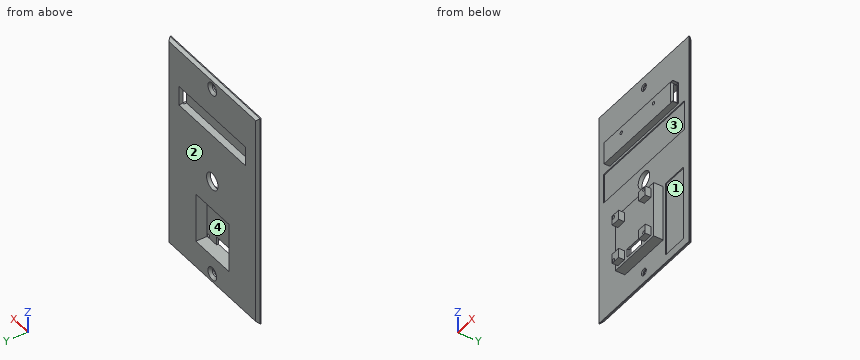
from build123d import *
from OCP.BRepFilletAPI import BRepFilletAPI_MakeChamfer

# Parameters (mm, degrees)
SKETCH2_W                = 69.35
SKETCH2_H                = 113.5
SKETCH2_R                = 1.85
BOSS_EXTRUDE3_DEPTH      = 2
SKETCH4_W                = 25.4
SKETCH4_H                = 26.1
CUT_EXTRUDE7_DEPTH       = 7.5
SKETCH16_W               = 29.414133621
SKETCH16_H               = 29.490350257
BOSS_EXTRUDE18_DEPTH     = 5
SKETCH17_W               = 25.4
SKETCH17_H               = 26.1
CUT_EXTRUDE8_DEPTH       = 4
SKETCH18_W               = 5
SKETCH18_H               = 5
BOSS_EXTRUDE24_DEPTH     = 4
SKETCH20_R               = 0.875
CUT_EXTRUDE10_DEPTH      = 4
SKETCH24_W               = 11
SKETCH24_H               = 4.5
CUT_EXTRUDE11_DEPTH      = 4
CHAMFER1_SIZE            = 1.5
CHAMFER1_SIZE2           = 1.258649447
SKETCH25_R               = 4.4
CUT_EXTRUDE12_DEPTH      = 4
SKETCH26_W               = 51.2
SKETCH26_H               = 10.3
CUT_EXTRUDE13_DEPTH      = 4
SKETCH27_W               = 52.651978828
SKETCH27_H               = 11.660574528
BOSS_EXTRUDE30_DEPTH     = 3
SKETCH30_W               = 51.2
SKETCH30_H               = 10.3
CUT_EXTRUDE14_DEPTH      = 3
SKETCH31_W               = 51.2
SKETCH31_H               = 10.3
BOSS_EXTRUDE31_DEPTH     = 1.5
SKETCH32_W               = 11.249454003
SKETCH32_H               = 2.603694337
CUT_EXTRUDE15_DEPTH      = 1.5
SKETCH33_W               = 1.5
SKETCH33_H               = 11.249454003
CUT_EXTRUDE16_DEPTH      = 1.5
SKETCH34_R               = 0.991075147
CUT_EXTRUDE17_DEPTH      = 1.5
SKETCH35_W               = 4.49763683
SKETCH35_H               = 1.113144729
CUT_EXTRUDE18_DEPTH      = 1.5
SKETCH36_W               = 62.277737466
SKETCH36_H               = 15.843958398
CUT_EXTRUDE19_DEPTH      = 0.5
SKETCH37_W               = 13.804637021
SKETCH37_H               = 39.531460558
CUT_EXTRUDE22_DEPTH      = 0.5
CHAMFER2_SIZE            = 1.5
CHAMFER2_SIZE2           = 1.258649447
CHAMFER3_SIZE            = 1.5
CHAMFER3_SIZE2           = 1.258649447
CUT_EXTRUDE23_DEPTH      = 67.821913509
CUT_EXTRUDE23_DEPTH_BACK = 67.821913509
SKETCH42_R               = 0.875


with BuildPart() as part:
    # Sketch2 → Boss-Extrude3 (new body)
    with BuildSketch(Plane(origin=(0, 0, 0), x_dir=(1, 0, 0), z_dir=(0, 1, 0))):
        Rectangle(SKETCH2_W, SKETCH2_H)
        with Locations(Location((0, 51.050462441, 0), (0, 0, 270))):
            Circle(SKETCH2_R, mode=Mode.SUBTRACT)
        with Locations(Location((0, -51.050462441, 0), (0, 0, 90))):
            Circle(SKETCH2_R, mode=Mode.SUBTRACT)
    extrude(amount=BOSS_EXTRUDE3_DEPTH)

    # Sketch4 → Cut-Extrude7 (cut)
    with BuildSketch(Plane(origin=(0, 2, 0), x_dir=(1, 0, 0), z_dir=(0, 1, 0))):
        with Locations((0, 28.375)):
            Rectangle(SKETCH4_W, SKETCH4_H)
    extrude(amount=-CUT_EXTRUDE7_DEPTH, mode=Mode.SUBTRACT)

    # Sketch16 → Boss-Extrude18 (add)
    with BuildSketch(Plane(origin=(0, 0, 0), x_dir=(-1, 0, 0), z_dir=(0, -1, 0))):
        with Locations((-0.116069165, 28.233366211)):
            Rectangle(SKETCH16_W, SKETCH16_H)
    extrude(amount=BOSS_EXTRUDE18_DEPTH)

    # Sketch17 → Cut-Extrude8 (cut)
    with BuildSketch(Plane(origin=(0, 0, 0), x_dir=(1, 0, 0), z_dir=(0, 1, 0))):
        with Locations((0, 28.375)):
            Rectangle(SKETCH17_W, SKETCH17_H)
    extrude(amount=-CUT_EXTRUDE8_DEPTH, mode=Mode.SUBTRACT)

    # Sketch18 → Boss-Extrude24 (add)
    with BuildSketch(Plane(origin=(0, -4, 0), x_dir=(1, 0, 0), z_dir=(0, 1, 0))):
        with Locations((-10.2, 38.925)):
            Rectangle(SKETCH18_W, SKETCH18_H)
        with Locations((10.2, 38.925)):
            Rectangle(SKETCH18_W, SKETCH18_H)
        with Locations((10.2, 17.825)):
            Rectangle(SKETCH18_W, SKETCH18_H)
        with Locations((-10.2, 17.825)):
            Rectangle(SKETCH18_W, SKETCH18_H)
    extrude(amount=-BOSS_EXTRUDE24_DEPTH)

    # Sketch20 → Cut-Extrude10 (cut)
    with BuildSketch(Plane(origin=(0, -8, 0), x_dir=(-1, 0, 0), z_dir=(0, -1, 0))):
        with Locations(Location((-11.659970213, 40.369100554, 0), (0, 0, 90))):
            Circle(SKETCH20_R)
        with Locations(Location((11.725608978, 40.361432855, 0), (0, 0, 270))):
            Circle(SKETCH20_R)
        with Locations(Location((11.725608978, 16.657728735, 0), (0, 0, 90))):
            Circle(SKETCH20_R)
        with Locations(Location((-11.659970213, 16.657728735, 0), (0, 0, 270))):
            Circle(SKETCH20_R)
    extrude(amount=-CUT_EXTRUDE10_DEPTH, mode=Mode.SUBTRACT)

    # Sketch24 → Cut-Extrude11 (cut)
    with BuildSketch(Plane(origin=(0, -4, 0), x_dir=(1, 0, 0), z_dir=(0, 1, 0))):
        with Locations((0, 39.175)):
            Rectangle(SKETCH24_W, SKETCH24_H)
    extrude(amount=-CUT_EXTRUDE11_DEPTH, mode=Mode.SUBTRACT)

    # Chamfer1: one chamfer whose edges measure the first distance from different faces: ONE call of the kernel's chamfer builder (chamfer() names one face for all edges)
    chamfer1_edges_1 = [part.edges().sort_by_distance(p)[0] for p in [
        (-34.675, 2, 0),
    ]]
    chamfer1_side_1 = [part.faces().sort_by_distance(p)[0] for p in [
        (-34.675, 1, 0),
    ]]
    chamfer1_edges_2 = [part.edges().sort_by_distance(p)[0] for p in [
        (0, 2, 56.75),
    ]]
    chamfer1_side_2 = [part.faces().sort_by_distance(p)[0] for p in [
        (0, 1, 56.75),
    ]]
    chamfer1_edges_3 = [part.edges().sort_by_distance(p)[0] for p in [
        (34.675, 2, 0),
    ]]
    chamfer1_side_3 = [part.faces().sort_by_distance(p)[0] for p in [
        (34.675, 1, 0),
    ]]
    chamfer1_edges_4 = [part.edges().sort_by_distance(p)[0] for p in [
        (0, 2, -56.75),
    ]]
    chamfer1_side_4 = [part.faces().sort_by_distance(p)[0] for p in [
        (0, 1, -56.75),
    ]]
    chamfer1 = BRepFilletAPI_MakeChamfer(part.part.solid().wrapped)
    for e in chamfer1_edges_1:
        chamfer1.Add(CHAMFER1_SIZE, CHAMFER1_SIZE2, e.wrapped, chamfer1_side_1[0].wrapped)  # the first distance lies on this face
    for e in chamfer1_edges_2:
        chamfer1.Add(CHAMFER1_SIZE, CHAMFER1_SIZE2, e.wrapped, chamfer1_side_2[0].wrapped)  # the first distance lies on this face
    for e in chamfer1_edges_3:
        chamfer1.Add(CHAMFER1_SIZE, CHAMFER1_SIZE2, e.wrapped, chamfer1_side_3[0].wrapped)  # the first distance lies on this face
    for e in chamfer1_edges_4:
        chamfer1.Add(CHAMFER1_SIZE, CHAMFER1_SIZE2, e.wrapped, chamfer1_side_4[0].wrapped)  # the first distance lies on this face
    add(Compound.cast(chamfer1.Shape()), mode=Mode.REPLACE)

    # Sketch25 → Cut-Extrude12 (cut)
    with BuildSketch(Plane(origin=(0, 2, 0), x_dir=(1, 0, 0), z_dir=(0, 1, 0))):
        with Locations(Location((0, 0, 0), (0, 0, 270))):
            Circle(SKETCH25_R)
    extrude(amount=-CUT_EXTRUDE12_DEPTH, mode=Mode.SUBTRACT)

    # Sketch26 → Cut-Extrude13 (cut)
    with BuildSketch(Plane(origin=(0, 2, 0), x_dir=(1, 0, 0), z_dir=(0, 1, 0))):
        with Locations((0.104035738, -30.584770495)):
            Rectangle(SKETCH26_W, SKETCH26_H)
    extrude(amount=-CUT_EXTRUDE13_DEPTH, mode=Mode.SUBTRACT)

    # Sketch27 → Boss-Extrude30 (add)
    with BuildSketch(Plane(origin=(0, 0, 0), x_dir=(-1, 0, 0), z_dir=(0, -1, 0))):
        with Locations((-0.102132054, -30.545281087)):
            Rectangle(SKETCH27_W, SKETCH27_H)
    extrude(amount=BOSS_EXTRUDE30_DEPTH)

    # Sketch30 → Cut-Extrude14 (cut)
    with BuildSketch(Plane(origin=(0, 0, 0), x_dir=(1, 0, 0), z_dir=(0, 1, 0))):
        with Locations((0.104035738, -30.584770495)):
            Rectangle(SKETCH30_W, SKETCH30_H)
    extrude(amount=-CUT_EXTRUDE14_DEPTH, mode=Mode.SUBTRACT)

    # Sketch31 → Boss-Extrude31 (add)
    with BuildSketch(Plane(origin=(0, -3, 0), x_dir=(-1, 0, 0), z_dir=(0, -1, 0))):
        with Locations((-0.104035738, -30.584770495)):
            Rectangle(SKETCH31_W, SKETCH31_H)
    extrude(amount=-BOSS_EXTRUDE31_DEPTH)

    # Sketch32 → Cut-Extrude15 (cut)
    with BuildSketch(Plane(origin=(26.428121468, 0, 0), x_dir=(0, 0, -1), z_dir=(1, 0, 0))):
        with Locations((-30.572653553, -1.487745374)):
            Rectangle(SKETCH32_W, SKETCH32_H)
    extrude(amount=-CUT_EXTRUDE15_DEPTH, mode=Mode.SUBTRACT)

    # Sketch33 → Cut-Extrude16 (cut)
    with BuildSketch(Plane(origin=(0, -2.789592542, 0), x_dir=(1, 0, 0), z_dir=(0, 1, 0))):
        with Locations((25.678121468, -30.572653553)):
            Rectangle(SKETCH33_W, SKETCH33_H)
    extrude(amount=-CUT_EXTRUDE16_DEPTH, mode=Mode.SUBTRACT)

    # Sketch34 → Cut-Extrude17 (cut)
    with BuildSketch(Plane.ZY.offset(26.22385736)):
        with Locations((34.622232322, -1.377930419)):
            Circle(SKETCH34_R)
    extrude(amount=-CUT_EXTRUDE17_DEPTH, mode=Mode.SUBTRACT)

    # Sketch35 → Cut-Extrude18 (cut)
    with BuildSketch(Plane.ZY.offset(26.22385736)):
        with Locations((33.35694274, -0.943427635)):
            Rectangle(SKETCH35_W, SKETCH35_H)
    extrude(amount=-CUT_EXTRUDE18_DEPTH, mode=Mode.SUBTRACT)

    # Sketch36 → Cut-Extrude19 (cut)
    with BuildSketch(Plane(origin=(0, 0, 0), x_dir=(-1, 0, 0), z_dir=(0, -1, 0))):
        with Locations((-0.078435438, -15.373345772)):
            Rectangle(SKETCH36_W, SKETCH36_H)
    extrude(amount=-CUT_EXTRUDE19_DEPTH, mode=Mode.SUBTRACT)

    # Sketch37 → Cut-Extrude22 (cut)
    with BuildSketch(Plane(origin=(0, 0, 0), x_dir=(-1, 0, 0), z_dir=(0, -1, 0))):
        with Locations((-23.687502159, 32.707577485)):
            Rectangle(SKETCH37_W, SKETCH37_H)
    extrude(amount=-CUT_EXTRUDE22_DEPTH, mode=Mode.SUBTRACT)

    # Chamfer2
    chamfer2_edges = [part.edges().sort_by_distance(p)[0] for p in [
        (0, 2, 52.900462441),
    ]]
    chamfer2_side = [part.faces().sort_by_distance(p)[0] for p in [
        (-32.120828655, 2, 0),
    ]]
    chamfer(chamfer2_edges, length=CHAMFER2_SIZE, length2=CHAMFER2_SIZE2, reference=chamfer2_side[0])

    # Chamfer3
    chamfer3_edges = [part.edges().sort_by_distance(p)[0] for p in [
        (0, 2, -52.900462441),
    ]]
    chamfer3_side = [part.faces().sort_by_distance(p)[0] for p in [
        (0, 2, 54.53001463),
    ]]
    chamfer(chamfer3_edges, length=CHAMFER3_SIZE, length2=CHAMFER3_SIZE2, reference=chamfer3_side[0])

    # Sketch42 → Cut-Extrude23 (cut, two sides: drawn at the far end of the back side and taken through both)
    with BuildSketch(Plane(origin=(0, -1.5, 0), x_dir=(1, 0, 0), z_dir=(0, 1, 0)).offset(-CUT_EXTRUDE23_DEPTH_BACK)):
        with Locations(Location((-12.995964262, -33.234770495, 0), (0, 0, 270))):
            Circle(SKETCH42_R)
        with Locations(Location((11.754035738, -33.234770495, 0), (0, 0, 270))):
            Circle(SKETCH42_R)
    extrude(amount=CUT_EXTRUDE23_DEPTH + CUT_EXTRUDE23_DEPTH_BACK, mode=Mode.SUBTRACT)


solid = part.part
Check sheet for the modelled part. Datum: model origin and axes. Units: mm. Face numbers are marked on the shaded views. A direction names the side the tool comes from. Give positions to 0.01 mm unless a question says otherwise; leave off trailing zeros. Write each loop counter-clockwise with the first axis right and the second up, starting at its lowest first coordinate (ties: lowest second). Pieces come first, ordered by that corner, then holes. Notation, with made-up numbers: (29.25, 76.5) -> (62.25, 76.5) arc R26 ccw to (62.25, 106.5) -> close; hole circle Ø4 at (82, 0). An arc over 180 degrees is marked (long way). Write item = value, one per line.
Item 1: Sectioned sample at C-C on z = 14.5. Record the boundary of the cut face in (x, y) (3 decimals), and give its area (3 significant figures).
Output:
outline = (-34.675, 0) -> (-31.06, 0) -> (-31.06, 0.5) -> (31.217, 0.5) -> (31.217, 0) -> (34.675, 0) -> (34.675, 0.5) -> (33.416, 2) -> (-33.416, 2) -> (-34.675, 0.5) -> close
area = 106 mm^2
Item 2: Scan lines: probe 1 along Z at (x, y) = (-13, -2.25) (3 decimals); probe 2 along Z at (x, y) = (-1, -3.25) (3 decimals); probe 3 along X at (y, z) = (-2.5, -16). Record each from-to range of solid material in increasing order. Write a range as from..to.
Output:
probe_1 = -42.979..-13.488, 24.715..32.36, 34.11..36.376
probe_2 = -42.979..-41.425, -15.325..-13.488
probe_3 = -14.59..-12.7, 12.7..14.82
Item 3: Sectioned sample at A-A on z = 0. Record the boundary of the cut face in (x, y) (3 decimals), and give its area (3 significant figures).
Output:
outline = (-34.675, 0) -> (-4.4, 0) -> (-4.4, 2) -> (-33.416, 2) -> (-34.675, 0.5) -> close; (4.4, 0) -> (34.675, 0) -> (34.675, 0.5) -> (33.416, 2) -> (4.4, 2) -> close
area = 119 mm^2
Item 4: Gauge pin test, flat ends, axial feed: pin 1 (1.6 mm diameter, centred on x = 25.5, y = -2, fed in from +Z); pin 2 (1.5 mm diameter, centred on x = 24, y = -2, fed in from -Z) (3 decimals); pin 3 (4.5 mm diameter, centred on x = 0, z = 51.05, fed in from -Y); pin 4 (23.5 mm diameter, centred on x = 2, z = -26.5, fed in from -Y). Record the tip position at first contact, or that the pin passes through.
Output:
pin_1 = 36.38
pin_2 = 24.715
pin_3 = 0
pin_4 = -8
Item 5: Sectioned sample at D-D on x = 0. Count the separate pieces of the cut face and the enclosed holes in it, and give its area (3 significant figures).
Output:
separate_pieces = 5
enclosed_holes = 0
area = 166 mm^2
Item 6: Sectioned sample at B-B on x = -27.5. Record the boundary of the cut face in (y, z).
Output:
outline = (0, -56.75) -> (0.5, -56.75) -> (2, -55.49) -> (2, 55.49) -> (0.5, 56.75) -> (0, 56.75) -> (0, 23.3) -> (0.5, 23.3) -> (0.5, 7.45) -> (0, 7.45) -> close
Item 7: Tool access check on the marked faces 3 and 4. Record the directions out of +Z, -Z, +X, -X, +Y, -Y that give a thin tool (end or side, any length) a straight path to the whole face; none if there is none.
Output:
face_3 = -Y
face_4 = +Y
Item 8: Release check for a two-part mould opening along Z. For the marked faces 1 and 2 record: +Z half, -Z half, draft (parallel to the pull), parting line (faces both ways), or undercut.
Output:
face_1 = undercut
face_2 = draft
